```python
from build123d import *

# Parameters (mm, degrees)
F0_W     = 204.8915475607
F0_H     = 180.7192862034
F1_DEPTH = 127
F2_R     = 25.4
F3_T     = -2.54


# Not quite as in the source:
# - a shell that OpenCascade refuses in one call is made with other operations: the cavity is built on its own and cut out


with BuildPart() as f1:
    # F0 (on Top) → F1 (new body)
    with BuildSketch(Plane.XY):
        Rectangle(F0_W, F0_H)
    extrude(amount=F1_DEPTH)

    # F2
    f2_edges = [f1.edges().sort_by_distance(p)[0] for p in [
        (-102.445774, -90.359643, 63.5),
        (102.445774, -90.359643, 63.5),
        (0, -90.359643, 0),
        (0, -90.359643, 127),
        (102.445774, 90.359643, 63.5),
        (102.445774, 0, 0),
        (102.445774, 0, 127),
        (0, 90.359643, 127),
        (-102.445774, 0, 127),
        (-102.445774, 90.359643, 63.5),
        (-102.445774, 0, 0),
        (0, 90.359643, 0),
    ]]
    fillet(f2_edges, radius=F2_R)

    # F3: a shell. OpenCascade refuses it in one call, so the cavity is built on its own and cut out:
    # the body offset inwards by the wall thickness, plus a prism from it out through each open face.
    f3_core = offset(f1.part, amount=F3_T, mode=Mode.PRIVATE)
    f3_exits = [f3_core.faces().sort_by_distance(p)[0] for p in [
        (0, 0, 124.46),
    ]]
    add(f3_core, mode=Mode.SUBTRACT)
    extrude(f3_exits, amount=-F3_T, mode=Mode.SUBTRACT)


solid = f1.part
```
Work out the finished part from the listing and answer in its coordinate system (mm). A direction names the side the tool comes from. Coordinates: 2 decimals unless noted, no trailing zeros. Loops run counter-clockwise (first coordinate to the right, second up) from the corner with the lowest first, then second, coordinate; pieces in that order, holes last. Notation, with made-up numbers: (64, -20.5) - (98, -20.5) arc R15 ccw to (98, 2.5) - close; hole circle Ø6 at (81, 25.25). An arc over 180 degrees is marked (long way). Use a Markdown table: item, result.
Item 1: Find section D-D, the plane x = -83. Determine the outline of the cut face in (y, z).
Evaluation:
| item | result |
|---|---|
| outline | (-89.65, 25.4) arc R24.69 ccw to (-64.96, 0.71) - (64.96, 0.71) arc R24.69 ccw to (89.65, 25.4) - (89.65, 101.6) arc R24.69 ccw to (64.96, 126.29) - (-64.96, 126.29) arc R24.69 ccw to (-89.65, 101.6) - close; hole (-87.03, 25.4) arc R22.07 ccw to (-64.96, 3.33) - (64.96, 3.33) arc R22.07 ccw to (87.03, 25.4) - (87.03, 101.6) arc R22.07 ccw to (64.96, 123.67) - (-64.96, 123.67) arc R22.07 ccw to (-87.03, 101.6) - close |
Item 2: The mould has two halves that part along Y. Classify faces 1 (the flat face through (-1, -90.36, 63)), 2 (the cylindrical face through (1.08, 83.12, 119.36)), 3 (the cylindrical face through (-93.387, 0.909, 9.414)): +Y half, -Y half, draft (parallel to the pull), parting line (faces both ways), or undercut.
Evaluation:
| item | result |
|---|---|
| face 1 | -Y half |
| face 2 | +Y half |
| face 3 | undercut |
Item 3: Given pin 1 Ø2 at (x, z) = (-18, 126) entering from +Y; pin 2 Ø0.8 at (x, z) = (22.5, 125.5) entering from -Y; pin 3 Ø5 at (x, y) = (-21.5, -11) entering from -Z; pin 4 Ø0.8 at (y, z) = (-18.5, 125.5) entering from +X, each flat-ended and moving along its own axis, determine where each tip first touches the part or whether it passes through.
Evaluation:
| item | result |
|---|---|
| pin 1 | stops at y = 74.84 |
| pin 2 | stops at y = -74.6 |
| pin 3 | stops at z = 0 |
| pin 4 | stops at x = 86.68 |
Item 4: Consider probe 1 along Y at (x, z) = (-5, 39); probe 2 along Y at (x, z) = (7.5, 103); probe 3 along X at (y, z) = (47, 80.5). Determine where each line is inside the solid, lowest interval first. Write a range as from..to.
Evaluation:
| item | result |
|---|---|
| probe 1 | y = -90.36..-87.82, 87.82..90.36 |
| probe 2 | y = -90.32..-87.78, 87.78..90.32 |
| probe 3 | x = -102.45..-99.91, 99.91..102.45 |
Item 5: Find section A-A, the plane z = 75. Determine the outline of the cut face in (x, y), and give its area (3 significant figures).
Evaluation:
| item | result |
|---|---|
| outline | (-102.45, -64.96) arc R25.4 ccw to (-77.05, -90.36) - (77.05, -90.36) arc R25.4 ccw to (102.45, -64.96) - (102.45, 64.96) arc R25.4 ccw to (77.05, 90.36) - (-77.05, 90.36) arc R25.4 ccw to (-102.45, 64.96) - close; hole (-99.91, -64.96) arc R22.86 ccw to (-77.05, -87.82) - (77.05, -87.82) arc R22.86 ccw to (99.91, -64.96) - (99.91, 64.96) arc R22.86 ccw to (77.05, 87.82) - (-77.05, 87.82) arc R22.86 ccw to (-99.91, 64.96) - close |
| area | 1,830 mm2 |
Item 6: Find section B-B, the plane y = -57. Determine the outline of the cut face in (x, z), and give its area (3 significant figures).
Evaluation:
| item | result |
|---|---|
| outline | (-102.45, 25.4) arc R25.4 ccw to (-77.05, 0) - (77.05, 0) arc R25.4 ccw to (102.45, 25.4) - (102.45, 101.6) arc R25.4 ccw to (77.05, 127) - (77.05, 124.46) arc R22.86 cw to (99.91, 101.6) - (99.91, 25.4) arc R22.86 cw to (77.05, 2.54) - (-77.05, 2.54) arc R22.86 cw to (-99.91, 25.4) - (-99.91, 101.6) arc R22.86 cw to (-77.05, 124.46) - (-77.05, 127) arc R25.4 ccw to (-102.45, 101.6) - close |
| area | 1,160 mm2 |
Item 7: Find section C-C, the plane x = -18.5. Determine the outline of the cut face in (y, z), and give its area (3 significant figures).
Evaluation:
| item | result |
|---|---|
| outline | (-90.36, 25.4) arc R25.4 ccw to (-64.96, 0) - (64.96, 0) arc R25.4 ccw to (90.36, 25.4) - (90.36, 101.6) arc R25.4 ccw to (64.96, 127) - (64.96, 124.46) arc R22.86 cw to (87.82, 101.6) - (87.82, 25.4) arc R22.86 cw to (64.96, 2.54) - (-64.96, 2.54) arc R22.86 cw to (-87.82, 25.4) - (-87.82, 101.6) arc R22.86 cw to (-64.96, 124.46) - (-64.96, 127) arc R25.4 ccw to (-90.36, 101.6) - close |
| area | 1,100 mm2 |
Item 8: For faces 4 (the flat face through (-1, 1, 2.54)), 5 (the cylindrical face through (-95.203, -82.722, 64.033)), 6 (the cylindrical face through (1.079, 81.301, 117.586)), determine the directions among +Z, -Z, +X, -X, +Y, -Y from which every point of the face is accessible in a straight line to the end or side of a thin tool.
Evaluation:
| item | result |
|---|---|
| face 4 | +Z |
| face 5 | +Z, -Z, -X, -Y |
| face 6 | none |
